Part model, mm, in its own coordinate system. Face numbers are marked on the shaded views. A direction names the side the tool comes from. Round coordinates to 2 decimals unless told otherwise and drop trailing zeros. Write each loop counter-clockwise with the first axis right and the second up, starting at its lowest first coordinate (ties: lowest second). Pieces come first, ordered by that corner, then holes. Notation, with made-up numbers: M 88.5,-14.5 L 119.5,-14.5 A13 ccw 119.5,-6.5 Z; hole C 73,83.5 d5. An arc over 180 degrees is marked long. Use one line per item in the form item = value. Start each with the question number.
Item 1: Mould opens along Z. For the marked faces 4, 5, 6 and 7 say: +Z half, -Z half, draft (parallel to the pull), parting line (faces both ways), or undercut.
Item 2: Cut at B-B, the plane x = 9. Give the cut face in (y, z).
Item 3: Flat gauge pins, fed straight in: pin 1 Ø18 at (x, y) = (-6, -12.5) entering from +Z; pin 2 Ø2 at (x, z) = (-9.5, -9) entering from -Y; pin 3 Ø3 at (x, z) = (-5, 0) entering from -Y. Where does each tip first touch, or does it go through?
Item 4: Cut at D-D, the plane z = -8. Give the cut face in (x, y), then the cut area to 3 significant figures.
Item 5: Probe L1, parallel to Y at x = -8.5, z = -51.5; L2, parallel to Z at x = 0, y = -18.75; L3, parallel to X at y = 14, z = -48. List the from-to ranges inside material, lowest first.
Item 6: Cut at A-A, the plane x = 0. Give the cut face in (y, z).
Item 7: Which spindle directions (+Z, -Z, +X, -X, +Y, -Y) get a long thin tool onto all of the face, cutting with end or side? Do the marked faces 1, 2 and 3. Say none if no direction does.
Item 8: Cut at C-C, the plane y = -17.5. Give the cut face in (x, z).
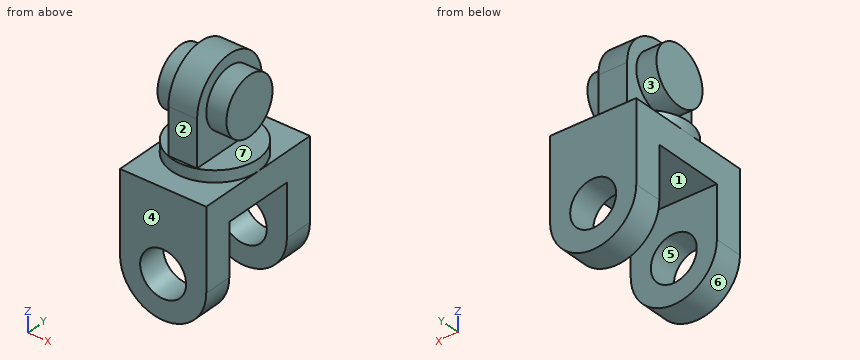
from build123d import *

# Parameters (mm, degrees)
SKETCH1_R           = 10
BOSS_EXTRUDE1_DEPTH = 12
BOSS_EXTRUDE2_DEPTH = 5
SKETCH3_R           = 15
BOSS_EXTRUDE3_DEPTH = 4
SKETCH5_W           = 30
SKETCH5_H           = 45
BOSS_EXTRUDE4_DEPTH = 10
BOSS_EXTRUDE5_START = 12.5
SKETCH7_R           = 8
BOSS_EXTRUDE5_DEPTH = 10
BOSS_EXTRUDE6_START = -12.5
SKETCH7_2_R         = 8
BOSS_EXTRUDE6_DEPTH = 10


with BuildPart() as part:
    # Sketch1 → Boss-Extrude1 (new body, symmetric)
    with BuildSketch(Plane(origin=(0, 0, 0), x_dir=(0, 0, -1), z_dir=(1, 0, 0))):
        Circle(SKETCH1_R)
    extrude(amount=BOSS_EXTRUDE1_DEPTH, both=True)

    # Sketch2 → Boss-Extrude2 (add, symmetric)
    with BuildSketch(Plane(origin=(0, 0, 0), x_dir=(0, 0, -1), z_dir=(1, 0, 0))):
        with BuildLine():
            Line((0, 14), (16, 14))
            Line((16, 14), (16, -14))
            Line((16, -14), (0, -14))
            ThreePointArc((0, -14), (-14, 0), (0, 14))
        make_face()
    extrude(amount=BOSS_EXTRUDE2_DEPTH, both=True)

    # Sketch3 → Boss-Extrude3 (add)
    with BuildSketch(Plane(origin=(0, 0, -16), x_dir=(-1, 0, 0), z_dir=(0, 0, -1))):
        Circle(SKETCH3_R)
    extrude(amount=BOSS_EXTRUDE3_DEPTH)

    # Sketch5 → Boss-Extrude4 (add)
    with BuildSketch(Plane(origin=(0, 0, -20), x_dir=(-1, 0, 0), z_dir=(0, 0, -1))):
        Rectangle(SKETCH5_W, SKETCH5_H)
    extrude(amount=BOSS_EXTRUDE4_DEPTH)

    # Sketch7 → Boss-Extrude5 (add)
    with BuildSketch(Plane(origin=(0, 0, 0), x_dir=(1, 0, 0), z_dir=(0, 1, 0)).offset(BOSS_EXTRUDE5_START)):
        with BuildLine():
            Line((-15, 30), (-15, 48))
            ThreePointArc((-15, 48), (0, 63), (15, 48))
            Line((15, 48), (15, 30))
            Line((15, 30), (-15, 30))
        make_face()
        with Locations((0, 48)):
            Circle(SKETCH7_R, mode=Mode.SUBTRACT)
    extrude(amount=BOSS_EXTRUDE5_DEPTH)

    # Sketch7<2> → Boss-Extrude6 (add)
    with BuildSketch(Plane(origin=(0, 0, 0), x_dir=(1, 0, 0), z_dir=(0, 1, 0)).offset(BOSS_EXTRUDE6_START)):
        with BuildLine():
            Line((-15, 30), (-15, 48))
            ThreePointArc((-15, 48), (0, 63), (15, 48))
            Line((15, 48), (15, 30))
            Line((15, 30), (-15, 30))
        make_face()
        with Locations((0, 48)):
            Circle(SKETCH7_2_R, mode=Mode.SUBTRACT)
    extrude(amount=-BOSS_EXTRUDE6_DEPTH)


solid = part.part
Model answer:
q1.face_4 = draft
q1.face_5 = undercut
q1.face_6 = -Z half
q1.face_7 = undercut
q2.outline = M -22.5,-60 L -12.5,-60 L -12.5,-30 L 12.5,-30 L 12.5,-60 L 22.5,-60 L 22.5,-20 L 12,-20 L 12,-16 L -12,-16 L -12,-20 L -22.5,-20 Z; C 0,0 d20
q3.pin_1 = 13.54
q3.pin_2 = -6
q3.pin_3 = -14
q4.outline = M -12,-6 L -5,-6 L -5,-14 L 5,-14 L 5,-6 L 12,-6 L 12,6 L 5,6 L 5,14 L -5,14 L -5,6 L -12,6 Z
q4.area = 448 mm²
q5.L1 = -22.5 to -12.5, 12.5 to 22.5
q5.L2 = -63 to -56, -40 to -20
q5.L3 = -15 to -8, 8 to 15
q6.outline = M -22.5,-63 L -12.5,-63 L -12.5,-56 L -22.5,-56 Z; M -22.5,-40 L -12.5,-40 L -12.5,-30 L 12.5,-30 L 12.5,-40 L 22.5,-40 L 22.5,-20 L 15,-20 L 15,-16 L 14,-16 L 14,0 A14 ccw -14,0 L -14,-16 L -15,-16 L -15,-20 L -22.5,-20 Z; M 12.5,-63 L 22.5,-63 L 22.5,-56 L 12.5,-56 Z
q7.face_1 = -Z, +X, -X
q7.face_2 = +Z, +X, -X, -Y
q7.face_3 = -X
q8.outline = M -15,-48 A15 ccw 15,-48 L 15,-20 L -15,-20 Z; hole C 0,-48 d16
